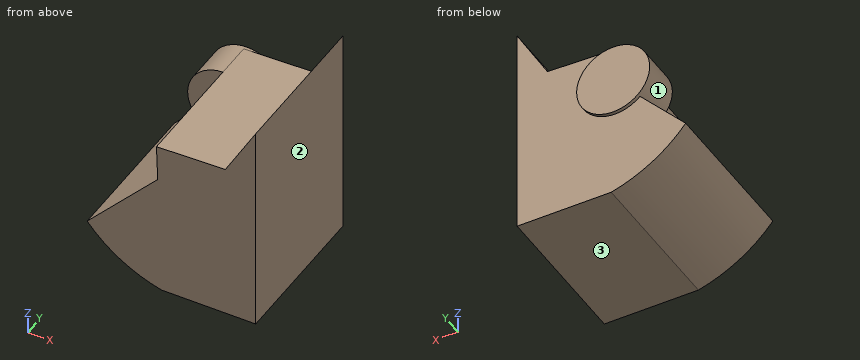
from build123d import *

# Parameters (mm, degrees)
BOSS_EXTRUDE1_DEPTH      = 223
BOSS_EXTRUDE2_DEPTH      = 5
BOSS_EXTRUDE2_DEPTH_BACK = 53
SKETCH3_R                = 53


with BuildPart() as part:
    # Sketch2 → Boss-Extrude1 (new body)
    with BuildSketch(Plane(origin=(0, 0, 0), x_dir=(1, 0, 0), z_dir=(0, 1, 0))):
        with BuildLine():
            Line((0, 0), (0, -311.121367585))
            Line((0, -311.121367585), (-44, -234.911132052))
            Line((-44, -234.911132052), (-143.9414944, -231.490942435))
            Line((-143.9414944, -231.490942435), (-142.128793904, -178.521950403))
            Line((-142.128793904, -178.521950403), (-244.505097616, -68.890328878))
            ThreePointArc((-244.505097616, -68.890328878), (-196.059281714, -25.695998193), (-136.456740169, 0))
            Line((-136.456740169, 0), (0, 0))
        make_face()
    extrude(amount=-BOSS_EXTRUDE1_DEPTH)

    # Sketch3 → Boss-Extrude2 (add, two sides: drawn at the far end of the back side and taken through both)
    with BuildSketch(Plane(origin=(0, 0, 0), x_dir=(1, 0, 0), z_dir=(0, 1, 0)).offset(-BOSS_EXTRUDE2_DEPTH_BACK)):
        with Locations(Location((-142.128793904, -178.521950403, 0), (0, 0, 270))):
            Circle(SKETCH3_R)
    extrude(amount=BOSS_EXTRUDE2_DEPTH + BOSS_EXTRUDE2_DEPTH_BACK)


solid = part.part
Read the model definition and answer for the solid it produces. Units are mm, in the model's axes. Face numbers are marked on the shaded views. Round coordinates to 2 decimals unless told otherwise and drop trailing zeros. Write each loop counter-clockwise with the first axis right and the second up, starting at its lowest first coordinate (ties: lowest second). Pieces come first, ordered by that corner, then holes. Notation, with made-up numbers: (-39.5, 69.25) - (-5.5, 69.25) arc R21 ccw to (-5.5, 107.25) - close; hole circle Ø7 at (70, 69). An arc over 180 degrees is marked (long way). One line per question, with ' | ' between items. Start each with the question number.
1. For a pull along Z with two mould halves and no side action, classify the marked faces 1, 2 and 3 as +Z half, -Z half, draft (parallel to the pull), parting line (faces both ways), or undercut.
2. Section B-B (x = -183.5) is taken. Determine the outline of the cut face in (y, z), and give its area (3 significant figures).
3. Each of these flat-tipped pins is pushed along its axis until it touches: pin 1 (6 mm diameter, centred on x = -163, z = 61.5, fed in from +Y); pin 2 (16 mm diameter, centred on x = -168.5, z = 185.5, fed in from -Y); pin 3 (1.5 mm diameter, centred on x = -206.5, y = -74, fed in from -Z). Where does it stop, or does it pass through?
4. Section D-D (x = -98) is taken. Determine the outline of the cut face in (y, z).
5. Section C-C (z = 130) is taken. Determine the outline of the cut face in (x, y), and give its area (3 significant figures).
6. Section A-A (y = -77.5) is taken. Determine the outline of the cut face in (x, z).
7. Find the intervals of material crossed by probe 1 along Y at (x, z) = (-174.5, 93.5); probe 2 along Z at (x, y) = (-44, -47.5); probe 3 along Y at (x, z) = (-152, 214), in increasing order. Write a range as [from, to].
Filled in:
1) face 1: undercut | face 2: draft | face 3: -Z half
2) outline: (-223, 18.31) - (0, 18.31) - (0, 134.22) - (-223, 134.22) - close; (-53, 145.39) - (5, 145.39) - (5, 211.65) - (-53, 211.65) - close | area: 29,700 mm²
3) pin 1: y = 0 | pin 2: y = -53 | pin 3: z = 32.28
4) outline: (-223, 0) - (0, 0) - (0, 149.17) - (5, 149.17) - (5, 207.88) - (0, 207.88) - (0, 233.06) - (-223, 233.06) - close
5) outline: (-187.44, -223) - (0, -223) - (0, 0) - (-120.81, 0) - (-120.81, 5) - (-163.45, 5) - (-163.45, 0) - (-187.44, 0) - close | area: 42,000 mm²
6) outline: (-244.51, 68.89) arc R203 ccw to (-136.46, 0) - (0, 0) - (0, 311.12) - (-44, 234.91) - (-143.94, 231.49) - (-142.13, 178.52) - close
7) probe 1: [-223, 0] | probe 2: [0, 234.91] | probe 3: [-53, 5]
